```python
from build123d import *

# Parameters (mm, degrees)
SKETCH1_W           = 62
SKETCH1_H           = 15
BOSS_EXTRUDE1_DEPTH = 2
SKETCH2_W           = 5
SKETCH2_H           = 5
BOSS_EXTRUDE2_DEPTH = 2


with BuildPart() as part:
    # Sketch1 → Boss-Extrude1 (new body)
    with BuildSketch(Plane(origin=(0, 0, 0), x_dir=(1, 0, 0), z_dir=(0, 1, 0))):
        with Locations((31, 7.5)):
            Rectangle(SKETCH1_W, SKETCH1_H)
    extrude(amount=BOSS_EXTRUDE1_DEPTH)

    # Sketch2 → Boss-Extrude2 (add)
    with BuildSketch(Plane(origin=(0, 2, 0), x_dir=(1, 0, 0), z_dir=(0, 1, 0))):
        with Locations((15.5, 7.5)):
            Rectangle(SKETCH2_W, SKETCH2_H)
        with Locations((46.5, 7.5)):
            Rectangle(SKETCH2_W, SKETCH2_H)
        Polygon((31, 2.5), (28.5, 2.5), (28.5, 12.5), (33.5, 12.5), (33.5, 2.5), align=None)
    extrude(amount=BOSS_EXTRUDE2_DEPTH)


solid = part.part
```
Source: CAD feature listing. Evaluate the final solid. Frame: model axes, mm. A direction names the side the tool comes from. Round coordinates to 2 decimals unless told otherwise and drop trailing zeros. Loops run counter-clockwise (first coordinate to the right, second up) from the corner with the lowest first, then second, coordinate; pieces in that order, holes last.
(1) Section query C-C (z = -7). Output: boundary loops of the cut face in (x, y), and give its area (3 significant figures).
From the geometry:
outline: (0, 0) - (62, 0) - (62, 2) - (49, 2) - (49, 4) - (44, 4) - (44, 2) - (33.5, 2) - (33.5, 4) - (28.5, 4) - (28.5, 2) - (18, 2) - (18, 4) - (13, 4) - (13, 2) - (0, 2) - close
area: 154 mm2
(2) Access query for faces 4 (the flat face through (18, 3, -7)), 5 (the flat face through (31, 3, -2.5)), 6 (the flat face through (15, 3, -5)). Directions: +Z, -Z, +X, -X, +Y, -Y. A direction counts if a zero-diameter tool reaches every point of the face in a straight line with its end or side. Return the directions, or none.
From the geometry:
face 4: +Z, -Z, +Y
face 5: +Z, +X, -X, +Y
face 6: +Z, -X, +Y
(3) Material intervals for probe 1 along X at (y, z) = (2.6, -5.25); probe 2 along Y at (x, z) = (42.5, -10); probe 3 along Z at (x, y) = (15.5, 3.15), sorted ascending.
From the geometry:
probe 1: x = 13 to 18, 28.5 to 33.5, 44 to 49
probe 2: y = 0 to 2
probe 3: z = -10 to -5
(4) Section query B-B (x = 47.5). Output: boundary loops of the cut face in (y, z), and give its area (3 significant figures).
From the geometry:
outline: (0, -15) - (2, -15) - (2, -10) - (4, -10) - (4, -5) - (2, -5) - (2, 0) - (0, 0) - close
area: 40.0 mm2
(5) Section query A-A (z = -11.5). Output: boundary loops of the cut face in (x, y), and give its area (3 significant figures).
From the geometry:
outline: (0, 0) - (62, 0) - (62, 2) - (33.5, 2) - (33.5, 4) - (28.5, 4) - (28.5, 2) - (0, 2) - close
area: 134 mm2
(6) Section query D-D (x = 35.5). Output: boundary loops of the cut face in (y, z).
From the geometry:
outline: (0, -15) - (2, -15) - (2, 0) - (0, 0) - close
(7) Pull-direction query (X, two-part tool) for faces 1 (the flat face through (49, 3, -7)), 2 (the flat face through (28.5, 3, -7)), 3 (the flat face through (15, 3, -10)); classes: +X half, -X half, draft (parallel to the pull), parting line (faces both ways), or undercut.
From the geometry:
face 1: +X half
face 2: undercut
face 3: draft
(8) Contact query for flat-ended pins moving along their axis: pin 1 Ø0.6 at (x, y) = (31.5, 3) entering from -Z; pin 2 Ø1.6 at (y, z) = (3, -8) entering from -X; pin 3 Ø2 at (y, z) = (3.5, -10) entering from +X. Output: stop coordinate, or through.
From the geometry:
pin 1: stops at z = -12.5
pin 2: stops at x = 13
pin 3: stops at x = 49
